Build history of the part. All positions in model axes, mm. Face numbers are marked on the shaded views. A direction names the side the tool comes from. Round coordinates to 2 decimals unless told otherwise and drop trailing zeros. Write each loop counter-clockwise with the first axis right and the second up, starting at its lowest first coordinate (ties: lowest second). Pieces come first, ordered by that corner, then holes. Notation, with made-up numbers: (78.5, 72.25) -> (101.5, 72.25) arc R25 cw to (101.5, 99.25) -> close; hole circle Ø10 at (-26.5, 83). An arc over 180 degrees is marked (long way). Return JSON: item names as keys, results as strings.
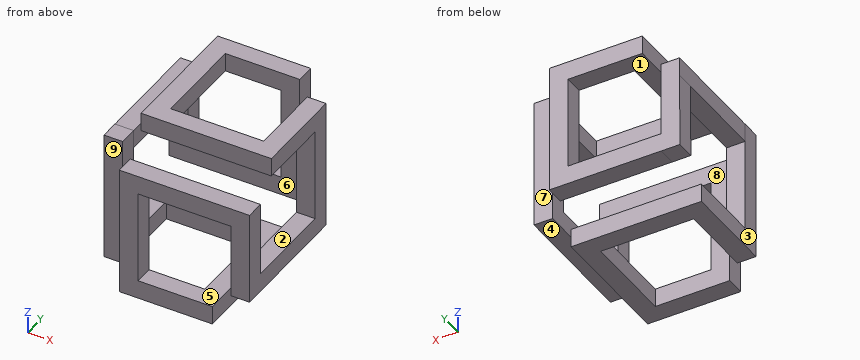
Autodesk Inventor part; units mm, degrees
ref_plane "YZ Plane" through (0, 0, 0) normal (1, 0, 0) x (0, 1, 0)
ref_plane "XZ Plane" through (0, 0, 0) normal (0, 1, 0) x (-1, 0, 0)
ref_plane "XY Plane" through (0, 0, 0) normal (0, 0, 1) x (1, 0, 0)
sketch "Sketch1" plane through (0, 0, 0) normal (0, 1, 0) x (-1, 0, 0)
  line L0 (0, 0) -> (0, -70)
  line L1 (0, -70) -> (70, -70)
  line L2 (70, -70) -> (70, 0)
  line L3 (70, 0) -> (0, 0)
  dimension "d0" = 70
  dimension "d1" = 70
  dimension "d2" = 70
extrude "Extrusion1" add sketch "Sketch1" along normal blind 10
sketch "Sketch2" plane through (0, 10, 0) normal (0, 1, 0) x (1, 0, 0)
  line L0 (-10, 10) -> (-10, 60)
  line L1 (-10, 60) -> (-60, 60)
  line L2 (-60, 60) -> (-60, 10)
  line L3 (-60, 10) -> (-10, 10)
  point P0 (0, 0)
  dimension "d7" = 50
  dimension "d8" = 50
  dimension "d9" = 50
extrude "Extrusion2" cut sketch "Sketch2" against normal blind 10
sketch "Sketch3" plane through (0, 10, 0) normal (0, 1, 0) x (1, 0, 0)
  line L0 (0, 70) -> (-70, 70)
  line L1 (0, 70) -> (0, 60)
  line L2 (0, 0) -> (0, 70)
  line L3 (0, 60) -> (-10, 60)
  line L4 (-10, 60) -> (-10, 70)
  dimension "d12" = 10
  dimension "d13" = 10
  dimension "d14" = 10
extrude "Extrusion3" cut sketch "Sketch3" against normal blind 10
sketch "Sketch4" plane through (0, 10, 0) normal (0, 1, 0) x (1, 0, 0)
  line L0 (-10, 60) -> (-60, 60)
  line L1 (-10, 60) -> (-10, 50)
  line L2 (-10, 60) -> (-10, 10)
  line L3 (-10, 50) -> (0, 50)
  line L4 (0, 0) -> (0, 60)
  line L5 (0, 50) -> (0, 60)
  line L6 (-10, 60) -> (0, 60)
  line L7 (0, 60) -> (-10, 60)
  dimension "d17" = 10
  dimension "d18" = 10
  dimension "d19" = 10
  dimension "d20" = 10
extrude "Extrusion4" cut sketch "Sketch4" against normal blind 10
sketch "Sketch5" plane through (0, 10, 0) normal (0, 1, 0) x (1, 0, 0)
  line L0 (-10, 60) -> (-10, 70)
  line L1 (-10, 60) -> (-10, 70)
  line L2 (-10, 70) -> (-20, 70)
  line L3 (-10, 70) -> (-70, 70)
  line L4 (-20, 70) -> (-20, 60)
  line L5 (-60, 60) -> (-10, 60)
  line L6 (-20, 60) -> (-10, 60)
  point P0 (0, 0)
  dimension "d23" = 10
  dimension "d24" = 10
  dimension "d25" = 10
  dimension "d26" = 10
extrude "Extrusion5" cut sketch "Sketch5" against normal blind 10
sketch "Sketch6" plane through (0, 10, 0) normal (0, 1, 0) x (1, 0, 0)
  line L0 (-10, 50) -> (0, 50)
  line L1 (-10, 50) -> (-10, 40)
  line L2 (-10, 40) -> (0, 40)
  line L3 (0, 0) -> (0, 50)
  line L4 (0, 40) -> (0, 50)
  line L5 (0, 50) -> (-10, 50)
  dimension "d29" = 10
  dimension "d30" = 10
  dimension "d31" = 10
  dimension "d32" = 10
extrude "Extrusion6" add sketch "Sketch6" along normal blind 70
sketch "Sketch7" plane through (0, 10, 0) normal (0, 1, 0) x (1, 0, 0)
  line L0 (-20, 60) -> (-30, 60)
  line L1 (-60, 60) -> (-20, 60)
  line L2 (-30, 60) -> (-30, 70)
  line L3 (-20, 70) -> (-70, 70)
  line L4 (-30, 70) -> (-20, 70)
  line L5 (-20, 70) -> (-20, 60)
  point P0 (0, 0)
  dimension "d35" = 10
  dimension "d36" = 10
  dimension "d37" = 10
  dimension "d38" = 10
extrude "Extrusion7" add sketch "Sketch7" along normal blind 60
sketch "Sketch8" plane through (0, 80, 0) normal (0, 1, 0) x (1, 0, 0)
  line L0 (0, 40) -> (-10, 40)
  line L1 (0, 40) -> (0, 50)
  line L2 (-10, 50) -> (0, 50)
  line L3 (0, 50) -> (-10, 50)
  line L4 (-10, 50) -> (-10, 40)
  line L5 (-10, 40) -> (0, 40)
  point P0 (0, 0)
  dimension "d41" = 10
  dimension "d42" = 10
  dimension "d43" = 10
  dimension "d44" = 10
extrude "Extrusion8" cut sketch "Sketch8" against normal blind 10
sketch "Sketch9" plane through (-10, 10, -40) normal (0, 0, 1) x (1, 0, 0)
  line L0 (10, 60) -> (0, 60)
  line L1 (0, 60) -> (0, 50)
  line L2 (0, 60) -> (0, -10)
  line L3 (0, 50) -> (10, 50)
  line L4 (10, -10) -> (10, 60)
  line L5 (10, 50) -> (10, 60)
  line L6 (10, 60) -> (0, 60)
  dimension "d47" = 10
  dimension "d48" = 10
  dimension "d49" = 10
  dimension "d50" = 10
extrude "Extrusion9" add sketch "Sketch9" along normal blind 60
sketch "Sketch10" plane through (-10, 60, -40) normal (0, -1, 0) x (1, 0, 0)
  line L0 (10, 60) -> (0, 60)
  line L1 (0, 60) -> (10, 60)
  line L2 (10, 60) -> (10, 50)
  line L3 (10, -10) -> (10, 60)
  line L4 (10, 50) -> (0, 50)
  line L5 (0, 60) -> (0, -10)
  line L6 (0, 50) -> (0, 60)
  point P0 (10, 40)
  dimension "d53" = 10
  dimension "d54" = 10
  dimension "d55" = 10
  dimension "d56" = 10
extrude "Extrusion10" add sketch "Sketch10" along normal blind 40
sketch "Sketch11" plane through (-10, 0, -10) normal (-1, 0, 0) x (0, 0, 1)
  line L0 (20, 20) -> (30, 20)
  line L1 (20, 20) -> (30, 20)
  line L2 (30, 20) -> (30, 30)
  line L3 (30, 70) -> (30, 20)
  line L4 (30, 30) -> (20, 30)
  line L5 (20, 60) -> (20, 20)
  line L6 (20, 30) -> (20, 20)
  point P0 (10, 0)
  dimension "d59" = 10
  dimension "d60" = 10
  dimension "d61" = 10
  dimension "d62" = 10
extrude "Extrusion11" add sketch "Sketch11" along normal blind 50
sketch "Sketch12" plane through (-30, 10, -70) normal (-1, 0, 0) x (0, 0, 1)
  line L0 (0, 60) -> (0, -10)
  line L1 (10, 60) -> (0, 60)
  line L2 (0, 60) -> (10, 60)
  line L3 (10, 60) -> (10, 50)
  line L4 (10, -10) -> (10, 60)
  line L5 (10, 50) -> (0, 50)
  line L6 (0, 50) -> (0, 60)
  line L7 (0, 60) -> (0, 55)
  point P0 (70, -10)
  dimension "d65" = 10
  dimension "d66" = 10
  dimension "d67" = 10
  dimension "d68" = 10
extrude "Extrusion12" add sketch "Sketch12" along normal blind 60
sketch "Sketch13" plane through (-90, 10, -70) normal (-1, 0, 0) x (0, 0, 1)
  point P0 (70, -10)
sketch "Sketch14" plane through (-30, 60, -70) normal (0, -1, 0) x (1, 0, 0)
  line L0 (10, 0) -> (-60, 0)
  line L1 (-60, 0) -> (-60, 10)
  line L2 (-60, 0) -> (-60, 10)
  line L3 (-60, 10) -> (-50, 10)
  line L4 (10, 10) -> (-60, 10)
  line L5 (-50, 10) -> (-50, 0)
  line L6 (-50, 0) -> (-60, 0)
  point P0 (30, 70)
  dimension "d71" = 10
  dimension "d72" = 10
  dimension "d73" = 10
  dimension "d74" = 10
extrude "Extrusion13" add sketch "Sketch14" along normal blind 40
sketch "Sketch15" plane through (-60, 0, -60) normal (0, 0, 1) x (1, 0, 0)
  line L0 (-20, 20) -> (-30, 20)
  line L1 (-30, 20) -> (-20, 20)
  line L2 (-20, 20) -> (-20, 30)
  line L3 (-20, 60) -> (-20, 20)
  line L4 (-20, 30) -> (-30, 30)
  line L5 (-30, 70) -> (-30, 20)
  line L6 (-30, 30) -> (-30, 20)
  point P0 (60, 0)
  dimension "d77" = 10
  dimension "d78" = 10
  dimension "d79" = 10
  dimension "d80" = 10
extrude "Extrusion14" add sketch "Sketch15" along normal blind 60
sketch "Sketch16" plane through (-60, 0, -10) normal (-1, 0, 0) x (0, 0, 1)
  point P0 (10, 0)
sketch "Sketch17" plane through (-60, 0, -10) normal (-1, 0, 0) x (0, 0, 1)
  line L0 (20, 20) -> (30, 20)
  line L1 (30, 20) -> (20, 20)
  line L2 (20, 20) -> (20, 30)
  line L3 (20, 60) -> (20, 20)
  line L4 (20, 30) -> (30, 30)
  line L5 (30, 70) -> (30, 20)
  line L6 (30, 30) -> (30, 20)
  point P0 (10, 0)
  dimension "d83" = 10
  dimension "d84" = 10
  dimension "d85" = 10
  dimension "d86" = 10
extrude "Extrusion15" add sketch "Sketch17" along normal blind 10
sketch "Sketch18" plane through (-90, 30, -60) normal (0, 1, 0) x (1, 0, 0)
  line L0 (90, -70) -> (20, -70)
  line L1 (20, -70) -> (20, -80)
  line L2 (20, -80) -> (30, -80)
  line L3 (30, -80) -> (30, -70)
  line L4 (30, -70) -> (20, -70)
  point P0 (90, -60)
  dimension "d89" = 10
  dimension "d90" = 10
  dimension "d91" = 10
  dimension "d92" = 10
extrude "Extrusion16" add sketch "Sketch18" along normal blind 60
sketch "Sketch19" plane through (-60, 30, 10) normal (1, 0, 0) x (0, 0, -1)
  line L0 (-10, 60) -> (0, 60)
  line L1 (0, 60) -> (0, 50)
  line L2 (0, 50) -> (-10, 50)
  line L3 (-10, 0) -> (-10, 60)
  line L4 (-10, 50) -> (-10, 60)
  point P0 (10, -30)
  dimension "d95" = 10
  dimension "d96" = 10
  dimension "d97" = 10
  dimension "d98" = 10
extrude "Extrusion17" add sketch "Sketch19" along normal blind 40
sketch "Sketch20" plane through (-90, 30, -60) normal (0, 1, 0) x (1, 0, 0)
  line L0 (0.0426, -60) -> (0, -50.0001)
  line L1 (0, 0) -> (0, -60)
  line L2 (0, -50.0001) -> (9.9999, -49.9575)
  line L3 (9.9999, -49.9575) -> (10.0425, -59.9574)
  line L4 (10.0425, -59.9574) -> (0.0426, -60)
  point P0 (90, -60)
  dimension "d101" = 10
  dimension "d102" = 10
  dimension "d103" = 10
  dimension "d104" = 10
extrude "Extrusion18" add sketch "Sketch20" along normal blind 60
sketch "Sketch21" plane through (-90, 30, -9.9999) normal (-0.0042561, 0, -0.9999909) x (-0.9999909, 0, 0.0042561)
  point P0 (-89.9566, -30)
sketch "Sketch22" plane through (-90, 30, -9.9999) normal (-0.0042561, 0, -0.9999909) x (-0.9999909, 0, 0.0042561)
  line L0 (0, 60) -> (-10, 60)
  line L1 (-10, 60) -> (0, 60)
  line L2 (0, 60) -> (0, 50)
  line L3 (0, 0) -> (0, 60)
  line L4 (0, 50) -> (-10, 50)
  line L5 (-10, 0) -> (-10, 60)
  line L6 (-10, 50) -> (-10, 60)
  point P0 (-89.9566, -30)
  dimension "d107" = 10
  dimension "d108" = 10
  dimension "d109" = 10
  dimension "d110" = 10
extrude "Extrusion19" add sketch "Sketch22" along normal blind 40
sketch "Sketch23" plane through (0, 60, 10) normal (0, 0, -1) x (-1, 0, 0)
  line L0 (70, 30) -> (20, 30)
  line L1 (20, 20) -> (20, 30)
  line L2 (20, 30) -> (20, 20)
  line L3 (20, 20) -> (30, 20)
  line L4 (60, 20) -> (20, 20)
  line L5 (30, 20) -> (30, 30)
  line L6 (30, 30) -> (20, 30)
  point P0 (0, -60)
  dimension "d113" = 10
  dimension "d114" = 10
  dimension "d115" = 10
  dimension "d116" = 10
extrude "Extrusion20" add sketch "Sketch23" along normal blind 60
sketch "Sketch24" plane through (-79.9575, 30, -0.0426) normal (0.9999909, 0, -0.0042561) x (-0.0042561, 0, -0.9999909)
  point P0 (-0.3829, -30)
sketch "Sketch25" plane through (-30, 80, 10) normal (-1, 0, 0) x (0, 0, 1)
  point P0 (-10, -80)
sketch "Sketch26" plane through (-30, 80, 10) normal (-1, 0, 0) x (0, 0, 1)
  line L0 (0, 10) -> (-60, 10)
  line L1 (-60, 10) -> (-60, 0)
  line L2 (-60, 0) -> (-50, 0)
  line L3 (0, 0) -> (-60, 0)
  line L4 (-50, 0) -> (-50, 10)
  line L5 (-50, 10) -> (-60, 10)
  point P0 (-10, -80)
  dimension "d119" = 10
  dimension "d120" = 10
  dimension "d121" = 10
  dimension "d122" = 10
extrude "Extrusion21" add sketch "Sketch26" along normal blind 60
properties part number "WeirdCube"
Q1. Wall check: L1, parallel to X at y = 34, z = 12; L2, parallel to Y at x = -48.5, z = 12. Give the ranges that are in metal, low to high.
Verdict:
{"L1": "x = -70 to -60, -10 to 0", "L2": "y = 20 to 30, 80 to 90"}
Q2. Saw through at C-C on x = -52. List the corners of the cut face in (y, z), then the cut area to 3 significant figures.
Verdict:
{"outline": "(0, -70) -> (10, -70) -> (10, -60) -> (0, -60) -> close; (0, -10) -> (10, -10) -> (10, 0) -> (0, 0) -> close; (20, 10) -> (30, 10) -> (30, 20) -> (20, 20) -> close; (60, -70) -> (70, -70) -> (70, -60) -> (60, -60) -> close; (80, -50) -> (90, -50) -> (90, -40) -> (80, -40) -> close; (80, 10) -> (90, 10) -> (90, 20) -> (80, 20) -> close", "area": "600 mm²"}
Q3. Saw through at B-B on y = 16.5. List the corners of the cut face in (x, z), then the cut area to 3 significant figures.
Verdict:
{"outline": "(-30, -70) -> (-20, -70) -> (-20, -60) -> (-30, -60) -> close; (-10, -50) -> (0, -50) -> (0, -40) -> (-10, -40) -> close", "area": "200 mm²"}
Q4. Saw through at A-A on x = -14. List the corners of the cut face in (y, z), then the cut area to 3 significant figures.
Verdict:
{"outline": "(0, -10) -> (10, -10) -> (10, 0) -> (0, 0) -> close; (20, 10) -> (30, 10) -> (30, 20) -> (20, 20) -> close", "area": "200 mm²"}
Q5. Two-plate mould, pull along Y, no slides. Class the marked faces 6, 7, 8 and 9: +Y half, -Y half, draft (parallel to the pull), parting line (faces both ways), or undercut.
Verdict:
{"face 6": "undercut", "face 7": "+Y half", "face 8": "undercut", "face 9": "-Y half"}
Q6. Saw through at D-D on y = 48. List the corners of the cut face in (x, z).
Verdict:
{"outline": "(-90, -70) -> (-80, -70) -> (-80, -60) -> (-90, -60) -> close; (-90, -10) -> (-80, -10.04) -> (-79.96, -0.04) -> (-89.96, 0) -> close; (-70, 10) -> (-60, 10) -> (-60, 20) -> (-70, 20) -> close; (-30, -70) -> (-20, -70) -> (-20, -60) -> (-30, -60) -> close; (-10, -50) -> (0, -50) -> (0, -40) -> (-10, -40) -> close; (-10, 10) -> (0, 10) -> (0, 20) -> (-10, 20) -> close"}
Q7. Pin check, flat tips, straight feed: pin 1 Ø6 at (y, z) = (25.5, -40.5) entering from -X; pin 2 Ø1.5 at (x, z) = (-27, -33) entering from -Y; pin 3 Ø3 at (x, y) = (-46.5, 2.5) entering from +Z; pin 4 Ø1.5 at (x, y) = (-48.5, 77.5) entering from -Z. Stop position of each tip, or through.
Verdict:
{"pin 1": "stops at x = -90", "pin 2": "stops at y = 80", "pin 3": "stops at z = 0", "pin 4": "passes through"}
Q8. 3-axis set-ups, long thin cutter, end or side, ignore diameter. For the marked faces 1, 2, 3, 4 and 5: which of +Z, -Z, +X, -X, +Y, -Y reach the whole face in a straight line?
Verdict:
{"face 1": "-X, -Y", "face 2": "+X", "face 3": "+Z, -Z, -X, -Y", "face 4": "-Z, +X, +Y, -Y", "face 5": "+X, +Y"}
